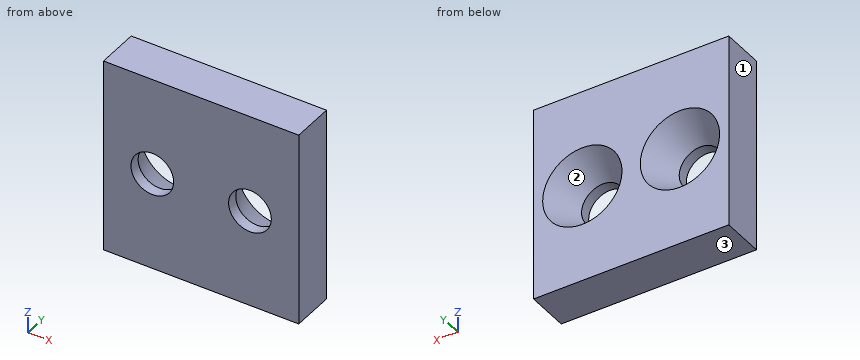
from build123d import *

# Parameters (mm, degrees)
SKETCH2_W           = 32
SKETCH2_H           = 32
SKETCH2_R           = 3.5
BOSS_EXTRUDE1_DEPTH = 7
CHAMFER2_SIZE       = 3
CHAMFER2_SIZE2      = 5.196152423
CHAMFER3_SIZE       = 3
CHAMFER3_SIZE2      = 5.196152423


with BuildPart() as part:
    # Sketch2 → Boss-Extrude1 (new body)
    with BuildSketch(Plane(origin=(0, 0, 0), x_dir=(1, 0, 0), z_dir=(0, 1, 0))):
        with Locations((16, 16)):
            Rectangle(SKETCH2_W, SKETCH2_H)
        with Locations((8, 16)):
            Circle(SKETCH2_R, mode=Mode.SUBTRACT)
        with Locations((24, 16)):
            Circle(SKETCH2_R, mode=Mode.SUBTRACT)
    extrude(amount=BOSS_EXTRUDE1_DEPTH)

    # Chamfer2
    chamfer2_edges = [part.edges().sort_by_distance(p)[0] for p in [
        (20.5, 7, -16),
    ]]
    chamfer2_side = [part.faces().sort_by_distance(p)[0] for p in [
        (16, 7, -16),
    ]]
    chamfer(chamfer2_edges, length=CHAMFER2_SIZE, length2=CHAMFER2_SIZE2, reference=chamfer2_side[0])

    # Chamfer3
    chamfer3_edges = [part.edges().sort_by_distance(p)[0] for p in [
        (4.5, 7, -16),
    ]]
    chamfer3_side = [part.faces().sort_by_distance(p)[0] for p in [
        (15.115857071, 7, -16),
    ]]
    chamfer(chamfer3_edges, length=CHAMFER3_SIZE, length2=CHAMFER3_SIZE2, reference=chamfer3_side[0])


solid = part.part
Geometry: final body of the model. Coordinates: model frame, mm. Face numbers are marked on the shaded views. Coordinates: 2 decimals unless noted, no trailing zeros. Order: outer loops, then holes, each group sorted by start corner. A loop starts at its lowest first (then second) coordinate and runs counter-clockwise, first axis right, second up.
(1) Section query C-C (y = 5). Return the cut outline in (x, z).
(2) First-contact query: pin 1 (9 mm diameter, centred on x = 24, z = -16, fed in from +Y). Flat tip, straight axial feed; report the tip coordinate or a pass-through.
(3) Material intervals for probe 1 along X at (y, z) = (0.75, -16); probe 2 along Z at (x, y) = (24, 0.9); probe 3 along X at (y, z) = (1.5, -19), sorted ascending.
(4) Section query B-B (z = -16). Return the cut outline in (x, y).
(5) Draft query along X for the marked faces 1, 2 and 3. Return one class per face: pulls with the +X half, pulls with the -X half, needs draft (parallel to the pull), parting line crosses it, or undercut.
(6) Section query A-A (x = 24). Return the cut outline in (y, z), plus the area to 3 significant figures.
(7) Section query D-D (y = 2.5). Return the cut outline in (x, z), plus the area to 3 significant figures.
Solution:
1. outline: (0, -32) - (32, -32) - (32, 0) - (0, 0) - close; hole circle Ø10.69 at (8, -16); hole circle Ø10.69 at (24, -16)
2. pin 1: stops at y = 3.54
3. probe 1: x = 0 to 4.5, 11.5 to 20.5, 27.5 to 32
3. probe 2: z = -32 to -19.5, -12.5 to 0
3. probe 3: x = 0 to 6.2, 9.8 to 22.2, 25.8 to 32
4. outline: (0, 0) - (4.5, 0) - (4.5, 1.8) - (1.5, 7) - (0, 7) - close; (11.5, 0) - (20.5, 0) - (20.5, 1.8) - (17.5, 7) - (14.5, 7) - (11.5, 1.8) - close; (27.5, 0) - (32, 0) - (32, 7) - (30.5, 7) - (27.5, 1.8) - close
5. face 1: pulls with the -X half
5. face 2: undercut
5. face 3: needs draft
6. outline: (0, -32) - (7, -32) - (7, -22.5) - (1.8, -19.5) - (0, -19.5) - close; (0, -12.5) - (1.8, -12.5) - (7, -9.5) - (7, 0) - (0, 0) - close
6. area: 159 mm2
7. outline: (0, -32) - (32, -32) - (32, 0) - (0, 0) - close; hole circle Ø7.8 at (8, -16); hole circle Ø7.8 at (24, -16)
7. area: 928 mm2
